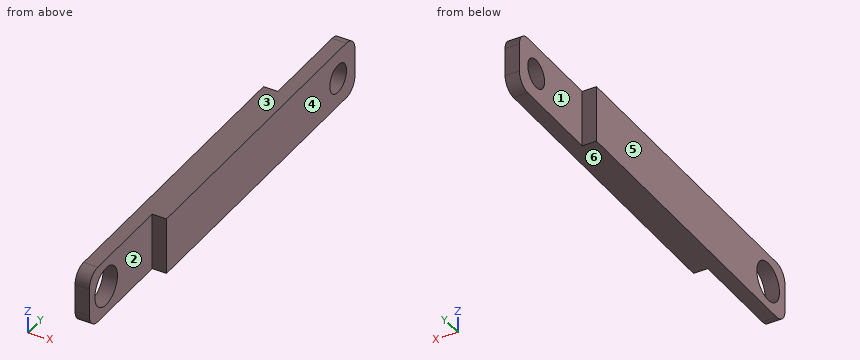
from build123d import *

# Parameters (mm, degrees)
SKETCH1_W           = 40
SKETCH1_H           = 300
BOSS_EXTRUDE1_DEPTH = 20
SKETCH2_W           = 40
SKETCH2_H           = 75
CUT_EXTRUDE1_DEPTH  = 10
SKETCH3_W           = 40
SKETCH3_H           = 75
CUT_EXTRUDE2_DEPTH  = 10
SKETCH4_R           = 13.5
CUT_EXTRUDE3_DEPTH  = 10
FILLET1_R           = 10
SKETCH5_R           = 10
CUT_EXTRUDE4_DEPTH  = 10


with BuildPart() as part:
    # Sketch1 → Boss-Extrude1 (new body)
    with BuildSketch(Plane(origin=(0, 0, 0), x_dir=(0, 0, -1), z_dir=(1, 0, 0))):
        Rectangle(SKETCH1_W, SKETCH1_H)
    extrude(amount=BOSS_EXTRUDE1_DEPTH)

    # Sketch2 → Cut-Extrude1 (cut)
    with BuildSketch(Plane.ZY):
        with Locations((0, 112.5)):
            Rectangle(SKETCH2_W, SKETCH2_H)
    extrude(amount=-CUT_EXTRUDE1_DEPTH, mode=Mode.SUBTRACT)

    # Sketch3 → Cut-Extrude2 (cut)
    with BuildSketch(Plane(origin=(20, 0, 0), x_dir=(0, 0, -1), z_dir=(1, 0, 0))):
        with Locations((0, -112.5)):
            Rectangle(SKETCH3_W, SKETCH3_H)
    extrude(amount=-CUT_EXTRUDE2_DEPTH, mode=Mode.SUBTRACT)

    # Sketch4 → Cut-Extrude3 (cut)
    with BuildSketch(Plane.ZY):
        with Locations((0, -130)):
            Circle(SKETCH4_R)
    extrude(amount=-CUT_EXTRUDE3_DEPTH, mode=Mode.SUBTRACT)

    # Fillet1
    fillet1_edges = [part.edges().sort_by_distance(p)[0] for p in [
        (5, -150, -20),
        (5, -150, 20),
        (15, 150, 20),
        (15, 150, -20),
    ]]
    fillet(fillet1_edges, radius=FILLET1_R)

    # Sketch5 → Cut-Extrude4 (cut)
    with BuildSketch(Plane(origin=(20, 0, 0), x_dir=(0, 0, -1), z_dir=(1, 0, 0))):
        with Locations((0, 130)):
            Circle(SKETCH5_R)
    extrude(amount=-CUT_EXTRUDE4_DEPTH, mode=Mode.SUBTRACT)


solid = part.part
CAD build for the part. Positions are in the model's coordinates, mm. Face numbers are marked on the shaded views. A direction names the side the tool comes from. Coordinates: 2 decimals unless noted, no trailing zeros. Write each loop counter-clockwise with the first axis right and the second up, starting at its lowest first coordinate (ties: lowest second). Pieces come first, ordered by that corner, then holes. Notation, with made-up numbers: (89, 7.5) - (144, 7.5) arc R20 ccw to (144, 45.5) - close; hole circle Ø6 at (8.25, 88). An arc over 180 degrees is marked (long way). Use a Markdown table: item, result. Add a question column.
Item 1: Band-saw the part on A-A, the plane x = 14.25. Give the cut face in (y, z), and give its area (3 significant figures).
Item 2: Mould opens along X. For the marked faces 4, 5 and 6 say: pulls with the +X half, pulls with the -X half, needs draft (parallel to the pull), parting line crosses it, or undercut.
Item 3: Band-saw the part on B-B, the plane y = -130. Give the cut face in (x, z), and give its area (3 significant figures).
Item 4: Band-saw the part on D-D, the plane y = 130. Give the cut face in (x, z), and give its area (3 significant figures).
Item 5: Band-saw the part on C-C, the plane z = 0. Give the cut face in (x, y).
Item 6: Flat gauge pins, fed straight in: pin 1 (3 mm diameter, centred on x = 5, z = 8.5, fed in from +Y); pin 2 (20 mm diameter, centred on y = 109.5, z = 8, fed in from -X). Where does each tip first touch, or does it go through?
Item 7: Drill centre lines: L1, parallel to Y at x = 14, z = 0; L2, parallel to Y at x = 7.25, z = 0; L3, parallel to X at y = -124, z = -15. Where is each one in solid material? Low to high. Write a range as from..to.
Item 8: 3-axis set-ups, long thin cutter, end or side, ignore diameter. For the marked faces 1, 2 and 3: which of +Z, -Z, +X, -X, +Y, -Y reach the whole face in a straight line?
Numbers:
| question | item | result |
|---|---|---|
| 1 | outline | (-75, -20) - (140, -20) arc R10 ccw to (150, -10) - (150, 10) arc R10 ccw to (140, 20) - (-75, 20) - close; hole circle Ø20 at (130, 0) |
| 1 | area | 8,640 mm2 |
| 2 | face 4 | pulls with the +X half |
| 2 | face 5 | pulls with the -X half |
| 2 | face 6 | needs draft |
| 3 | outline | (0, -20) - (10, -20) - (10, -13.5) - (0, -13.5) - close; (0, 13.5) - (10, 13.5) - (10, 20) - (0, 20) - close |
| 3 | area | 130 mm2 |
| 4 | outline | (10, -20) - (20, -20) - (20, -10) - (10, -10) - close; (10, 10) - (20, 10) - (20, 20) - (10, 20) - close |
| 4 | area | 200 mm2 |
| 5 | outline | (0, -150) - (10, -150) - (10, -143.5) - (0, -143.5) - close; (0, -116.5) - (10, -116.5) - (10, -75) - (20, -75) - (20, 120) - (10, 120) - (10, 75) - (0, 75) - close; (10, 140) - (20, 140) - (20, 150) - (10, 150) - close |
| 6 | pin 1 | y = 75 |
| 6 | pin 2 | x = 10 |
| 7 | L1 | -75..120, 140..150 |
| 7 | L2 | -150..-143.5, -116.5..75 |
| 7 | L3 | 0..10 |
| 8 | face 1 | +Z, -Z, -X, +Y |
| 8 | face 2 | +Z, -Z, +X, -Y |
| 8 | face 3 | +Z, +X, -X, +Y, -Y |
